Geometry check sheet. Reference: drawing and pictorial views, mm from the part's lowest x, y, z. A direction names the side the tool comes from. Round coordinates to 2 decimals unless told otherwise and drop trailing zeros. Loops run counter-clockwise (first coordinate to the right, second up) from the corner with the lowest first, then second, coordinate; pieces in that order, holes last. Notation, with made-up numbers: (-3.5, 74.25) -> (7.5, 74.25) arc R7 ccw to (7.5, 84.25) -> close; hole circle Ø7 at (63, -12.75). An arc over 180 degrees is marked (long way). Use one line per item in the form item = value.
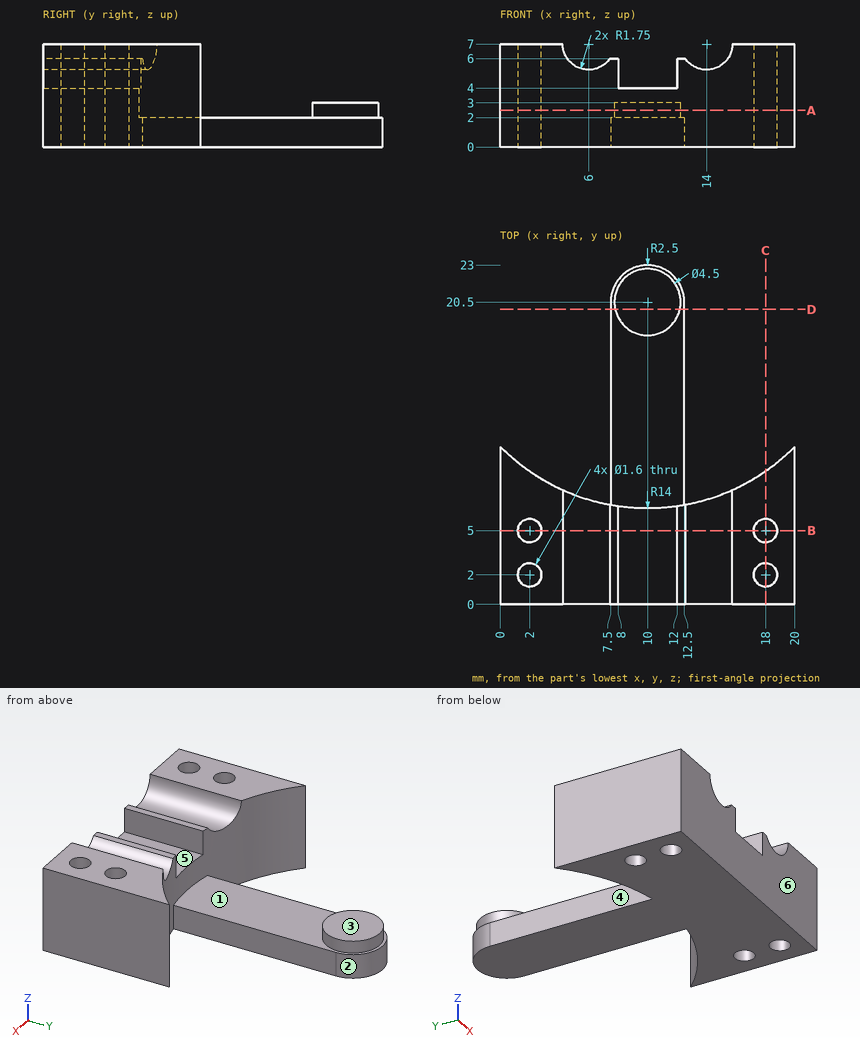
1. Section check C-C (x = 18). Record the boundary of the cut face in (y, z), then the cut area to 3 significant figures.
Return value:
outline = (0, 0) -> (1.2, 0) -> (1.2, 7) -> (0, 7) -> close; (2.8, 0) -> (4.2, 0) -> (4.2, 7) -> (2.8, 7) -> close; (5.8, 0) -> (9.01, 0) -> (9.01, 7) -> (5.8, 7) -> close
area = 40.7 mm2
2. Mould release check, pull along Y, two halves, no side actions. Record for the marked faces 1, 2 and 3: released by +Y, released by -Y, zero draft, split by the parting line, or undercut.
Return value:
face_1 = undercut
face_2 = released by +Y
face_3 = zero draft
3. Section check B-B (y = 5). Record the boundary of the cut face in (x, z), then the cut area to 3 significant figures.
Return value:
outline = (0, 0) -> (1.2, 0) -> (1.2, 7) -> (0, 7) -> close; (2.8, 0) -> (17.2, 0) -> (17.2, 7) -> (15.75, 7) arc R1.75 cw to (12.56, 6) -> (12, 6) -> (12, 4) -> (8, 4) -> (8, 6) -> (7.44, 6) arc R1.75 cw to (4.25, 7) -> (2.8, 7) -> close; (18.8, 0) -> (20, 0) -> (20, 7) -> (18.8, 7) -> close
area = 95.3 mm2
4. Section check D-D (y = 20). Record the boundary of the cut face in (x, z), then the cut area to 3 significant figures.
Return value:
outline = (7.5, 0) -> (12.5, 0) -> (12.5, 2) -> (12.19, 2) -> (12.19, 3) -> (7.81, 3) -> (7.81, 2) -> (7.5, 2) -> close
area = 14.4 mm2
5. Material ranges on line 1 along Y through (x, z) = (2, 2.5); line 2 along Y through (x, z) = (1.5, 5.75); line 3 along X through (y, z) = (12.75, 0.75), recorded low to high.
Return value:
line_1 = 0 to 1.2, 2.8 to 4.2, 5.8 to 9.01
line_2 = 0 to 1.38, 2.62 to 4.38, 5.62 to 9.38
line_3 = 7.5 to 12.5
6. Gauge pin test, flat ends, axial feed: pin 1 (3.5 mm diameter, centred on x = 9, y = 20.5, fed in from +Z); pin 2 (0.6 mm diameter, centred on x = 12, y = 2, fed in from +Z); pin 3 (5.5 mm diameter, centred on x = 9.5, y = 11.5, fed in from +Z). Record the tip position at first contact, or that the pin passes through.
Return value:
pin_1 = 3
pin_2 = 6
pin_3 = 2
7. Section check A-A (z = 2.5). Record the boundary of the cut face in (x, y).
Return value:
outline = (0, 0) -> (20, 0) -> (20, 10.7) arc R14 cw to (0, 10.7) -> close; circle Ø4.5 at (10, 20.5); hole circle Ø1.6 at (2, 2); hole circle Ø1.6 at (2, 5); hole circle Ø1.6 at (18, 2); hole circle Ø1.6 at (18, 5)
8. Tool access check on the marked faces 4, 5 and 6. Record the directions out of +Z, -Z, +X, -X, +Y, -Y that give a thin tool (end or side, any length) a straight path to the whole face; none if there is none.
Return value:
face_4 = +Z, -Z, +Y
face_5 = +Z, +Y, -Y
face_6 = +Z, -Z, +X, -X, -Y
